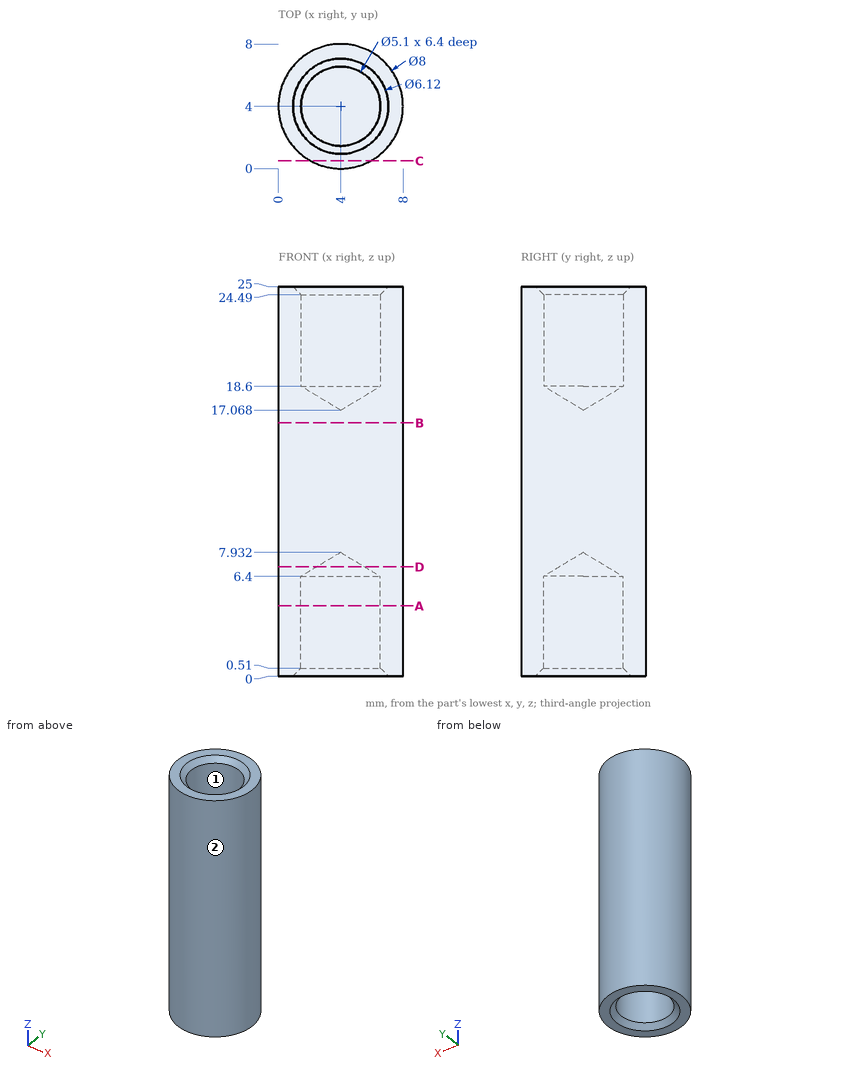
Drawing for the job (mm, zero at the part's lowest x, y, z). Round coordinates to 2 decimals unless told otherwise and drop trailing zeros. Loops run counter-clockwise (first coordinate to the right, second up) from the corner with the lowest first, then second, coordinate; pieces in that order, holes last.
1. Drop flat-ended pins along their axis: P1, Ø1, axis at x = 6.5, z = 16.5, coming from the +Y side; P2, Ø1.5, axis at x = 2, z = 19, coming from the +Y side. Give the stop position or say it passes through.
Check values:
P1: stops at y = 7.46
P2: stops at y = 7.8
2. Wall check: probe 1 along Y at (x, z) = (4, 4); probe 2 along Y at (x, z) = (2.25, 22) (1 decimal); probe 3 along X at (y, z) = (2, 21.5) (1 decimal). Give the ranges that are in metal, low to high.
Check values:
probe 1: y = 0 to 1.45, 6.55 to 8
probe 2: y = 0.4 to 2.1, 5.9 to 7.6
probe 3: x = 0.5 to 2.4, 5.6 to 7.5
3. Band-saw the part on B-B, the plane z = 16.25. List the corners of the cut face in (x, y), and give its area (3 significant figures).
Check values:
outline: circle Ø8 at (4, 4)
area: 50.3 mm2
4. Mould opens along X. For the marked faces 1 and 2 say: +X half, -X half, draft (parallel to the pull), parting line (faces both ways), or undercut.
Check values:
face 1: undercut
face 2: parting line
5. Band-saw the part on A-A, the plane z = 4.5. List the corners of the cut face in (x, y).
Check values:
outline: circle Ø8 at (4, 4); hole circle Ø5.1 at (4, 4)
6. Band-saw the part on D-D, the plane z = 7. List the corners of the cut face in (x, y).
Check values:
outline: circle Ø8 at (4, 4); hole circle Ø3.1 at (4, 4)
7. Band-saw the part on C-C, the plane y = 0.5. List the corners of the cut face in (x, z), and give its area (3 significant figures).
Check values:
outline: (2.06, 0) - (5.94, 0) - (5.94, 25) - (2.06, 25) - close
area: 96.8 mm2
